Read the model definition and answer for the solid it produces. Units are mm, in the model's axes. A direction names the side the tool comes from. Give positions to 0.01 mm unless a question says otherwise; leave off trailing zeros. Write each loop counter-clockwise with the first axis right and the second up, starting at its lowest first coordinate (ties: lowest second). Pieces come first, ordered by that corner, then holes. Notation, with made-up numbers: (44.25, 6.5) -> (85.25, 6.5) arc R32 ccw to (85.25, 39.5) -> close; hole circle Ø6 at (57.5, -13). An arc over 180 degrees is marked (long way). Write item = value, one per line.
from build123d import *

# Parameters (mm, degrees)
F1_DEPTH  = 38
F2_W      = 324
F2_H      = 38
F3_DEPTH  = 38
F4_W      = 38
F4_H      = 38
F5_DEPTH  = 324
F7_DEPTH  = 38
F8_T      = -2.5
F9_R      = 4
F10_DEPTH = 200.001


with BuildPart() as f1:
    # F0 (on Front) → F1 (new body)
    with BuildSketch(Plane.XZ):
        Polygon((0, 200), (0, 0), (38, 0), (38, 162), (1162, 162), (1162, 0), (1200, 0), (1200, 200), (1162, 200), (38, 200), align=None)
    extrude(amount=F1_DEPTH)

    # F2 (on face) → F3 (join)
    with BuildSketch(Plane(origin=(0, 0, 0), x_dir=(0, -1, 0), z_dir=(-1, 0, 0))):
        with Locations((-162, 181)):
            Rectangle(F2_W, F2_H)
    extrude(amount=-F3_DEPTH)

    # F4 (on face) → F5 (join)
    with BuildSketch(Plane(origin=(0, 0, 0), x_dir=(-1, 0, 0), z_dir=(0, 1, 0))):
        with Locations((-1181, 181)):
            Rectangle(F4_W, F4_H)
    extrude(amount=F5_DEPTH)

    # F6 (on face) → F7 (join)
    with BuildSketch(Plane(origin=(0, 324, 0), x_dir=(-1, 0, 0), z_dir=(0, 1, 0))):
        Polygon((-1162, 200), (-1200, 200), (-1200, 162), (-1200, 0), (-1162, 0), (-1162, 162), (-38, 162), (-38, 0), (0, 0), (0, 162), (0, 200), (-38, 200), align=None)
    extrude(amount=F7_DEPTH)

    # F8
    f8_openings = [f1.faces().sort_by_distance(p)[0] for p in [
        (19, 343, 0),
        (19, -19, 0),
        (1181, -19, 0),
        (1181, 343, 0),
    ]]
    offset(amount=F8_T, openings=f8_openings, kind=Kind.INTERSECTION)

    # F9 (on face) → F10 (cut, through all)
    with BuildSketch(Plane.XY.offset(200)):
        with BuildLine():
            ThreePointArc((215.25, 347), (214.0784271247, 349.8284271247), (211.25, 351))
            Line((211.25, 351), (211.25, 347))
            Line((211.25, 347), (215.25, 347))
        make_face()
        with BuildLine():
            ThreePointArc((461.75, 347), (457.75, 351), (453.75, 347))
            ThreePointArc((453.75, 347), (457.75, 343), (461.75, 347))
        make_face()
        with BuildLine():
            Line((211.25, 347), (211.25, 351))
            ThreePointArc((211.25, 351), (208.4215728753, 344.1715728753), (215.25, 347))
            Line((215.25, 347), (211.25, 347))
        make_face()
        with Locations((988.75, 347)):
            Circle(F9_R)
        with Locations((742.25, 347)):
            Circle(F9_R)
        with Locations((211.25, -23)):
            Circle(F9_R)
        with Locations((457.75, -23)):
            Circle(F9_R)
        with Locations((742.25, -23)):
            Circle(F9_R)
        with Locations((988.75, -23)):
            Circle(F9_R)
        with BuildLine():
            ThreePointArc((11, 81), (15, 77), (19, 81))
            ThreePointArc((19, 81), (15, 85), (11, 81))
        make_face()
        with Locations((15, 243)):
            Circle(F9_R)
        with Locations((1185, 243)):
            Circle(F9_R)
        with Locations((1185, 81)):
            Circle(F9_R)
    extrude(amount=-F10_DEPTH, mode=Mode.SUBTRACT)


solid = f1.part
(1) A tool of negligible diameter and unlimited length cuts with its end or side. For faces 1 (the flat face through (608, 343, 164.5)), 2 (the flat face through (1164.5, 343, 81)), 3 (the flat face through (1181, 160, 162)), from which of +Z, -Z, +X, -X, +Y, -Y can it reach the whole face along a straight path? Write none if from no direction.
Checks:
face_1 = none
face_2 = -Z
face_3 = -Z, +X, -X
(2) The part is cut by section A-A on y = 143. Determine the outline of the cut face in (x, z), plus the area to 3 significant figures.
Checks:
outline = (0, 162) -> (38, 162) -> (38, 200) -> (0, 200) -> close; (1162, 162) -> (1200, 162) -> (1200, 200) -> (1162, 200) -> close; hole (2.5, 164.5) -> (35.5, 164.5) -> (35.5, 197.5) -> (2.5, 197.5) -> close; hole (1164.5, 164.5) -> (1197.5, 164.5) -> (1197.5, 197.5) -> (1164.5, 197.5) -> close
area = 710 mm²
(3) The part is cut by section C-C on x = 92.5. Determine the outline of the cut face in (y, z).
Checks:
outline = (-38, 162) -> (0, 162) -> (0, 200) -> (-38, 200) -> close; (324, 162) -> (362, 162) -> (362, 200) -> (324, 200) -> close; hole (-35.5, 164.5) -> (-2.5, 164.5) -> (-2.5, 197.5) -> (-35.5, 197.5) -> close; hole (326.5, 164.5) -> (359.5, 164.5) -> (359.5, 197.5) -> (326.5, 197.5) -> close
(4) For a pull along Z with two mould halves and no side action, classify faces 4 (the flat face through (1164.5, 160, 181)), 5 (the flat face through (1181, 0, 82)), 6 (the flat face through (608, 343, 162)) as released by +Z, released by -Z, zero draft, split by the parting line, or undercut.
Checks:
face_4 = undercut
face_5 = zero draft
face_6 = released by -Z
(5) Consider L1, parallel to Y at x = 370, z = 184.5; L2, parallel to Y at x = 742.25, z = 198; L3, parallel to X at y = 261, z = 179.5. Determine where each line is inside the solid, lowest interval first.
Checks:
L1 = -38 to -35.5, -2.5 to 0, 324 to 326.5, 359.5 to 362
L2 = -38 to -27, -19 to 0, 324 to 343, 351 to 362
L3 = 0 to 2.5, 35.5 to 38, 1162 to 1164.5, 1197.5 to 1200
(6) Given P1, Ø10, axis at y = -15.5, z = 98, coming from the -X side; P2, Ø6.5, axis at x = 457.75, y = 347, coming from the +Z side, each flat-ended and moving along its own axis, determine where each tip first touches the part or whether it passes through.
Checks:
P1 = 0
P2 = through
(7) The part is cut by section B-B on z = 110. Count the separate pieces of the cut face and the enclosed holes in it, plus the area to 3 significant figures.
Checks:
separate_pieces = 4
enclosed_holes = 4
area = 1,420 mm²
